Check sheet for the modelled part. Datum: model origin and axes. Units: mm. Face numbers are marked on the shaded views. A direction names the side the tool comes from. Round coordinates to 2 decimals unless told otherwise and drop trailing zeros. Order: outer loops, then holes, each group sorted by start corner. A loop starts at its lowest first (then second) coordinate and runs counter-clockwise, first axis right, second up.
Q1. Cross-section at A-A on z = 43.5. Record the cut outline in (x, y), then the cut area to 3 significant figures.
Q2. Scan lines: probe 1 along X at (y, z) = (-35, 46.5); probe 2 along Y at (x, z) = (-42, 41.25); probe 3 along X at (y, z) = (-59.5, 40.5). Record each from-to range of solid material in increasing order.
Q3. Cross-section at D-D on z = 49. Record the cut outline in (x, y).
Q4. Cross-section at C-C on y = -49. Record the cut outline in (x, z).
Q5. Set-up check for the marked faces 1 and 2: record each of +Z, -Z, +X, -X, +Y, -Y from which the full face is reachable in a straight line by a thin tool's end or side.
Q6. Cross-section at B-B on x = -55. Record the cut outline in (y, z), then the cut area to 3 significant figures.
Q7. Depth check by flat-ended pin: P1, Ø1, axis at x = -44, y = -26.5, coming from the -Z side; P2, Ø4, axis at x = -65.5, z = 44, coming from the -Y side; P3, Ø3, axis at x = -36, z = 42.5, coming from the -Y side. Enter the tip coordinate at first touch or a pass-through.
Q8. Mould release check, pull along X, two halves, no side actions. Record for the marked faces 3, 4, 5 and 6: +X half, -X half, draft (parallel to the pull), parting line (faces both ways), or undercut.
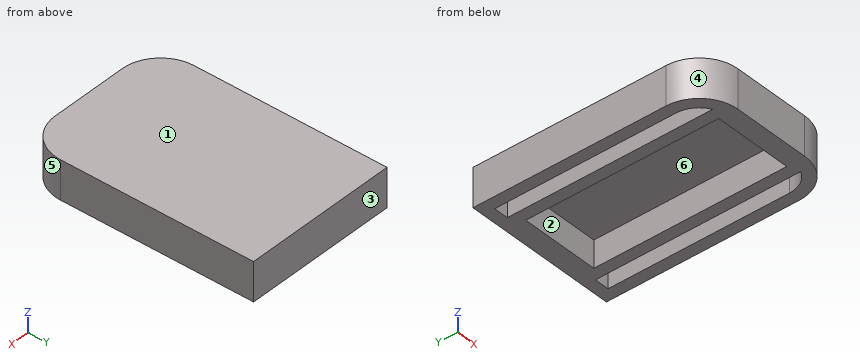
from build123d import *

# Parameters (mm, degrees)
SALIENTE_EXTRUIR1_DEPTH      = 50
CROQUIS2_W                   = 40
CROQUIS2_H                   = 50
SALIENTE_EXTRUIR2_DEPTH      = 60
SALIENTE_EXTRUIR2_DEPTH_BACK = 31
REDONDEO1_R                  = 10
REDONDEO2_R                  = 10
CORTAR_EXTRUIR1_DEPTH        = 74
VACIADO1_T                   = -3
CROQUIS4_W                   = 26.4
CROQUIS4_H                   = 56
CROQUIS4_W_2                 = 20.4
CROQUIS4_H_2                 = 50
SALIENTE_EXTRUIR3_DEPTH      = 7


with BuildPart() as part:
    # Croquis1 → Saliente-Extruir1 (new body)
    with BuildSketch(Plane.XY):
        with BuildLine():
            Line((-80.606796451, 54.173553719), (-40.606796451, 54.173553719))
            ThreePointArc((-40.606796451, 54.173553719), (-33.53572864, 51.244621531), (-30.606796451, 44.173553719))
            Line((-30.606796451, 44.173553719), (-30.606796451, 4.173553719))
            ThreePointArc((-30.606796451, 4.173553719), (-33.53572864, -2.897514093), (-40.606796451, -5.826446281))
            Line((-40.606796451, -5.826446281), (-80.606796451, -5.826446281))
            ThreePointArc((-80.606796451, -5.826446281), (-87.677864263, -2.897514093), (-90.606796451, 4.173553719))
            Line((-90.606796451, 4.173553719), (-90.606796451, 44.173553719))
            ThreePointArc((-90.606796451, 44.173553719), (-87.677864263, 51.244621531), (-80.606796451, 54.173553719))
        make_face()
    extrude(amount=SALIENTE_EXTRUIR1_DEPTH)

    # Croquis2 → Saliente-Extruir2 (add, two sides)
    with BuildSketch(Plane.XZ.offset(5.826446281)) as saliente_extruir2_sk:
        with Locations((-50.606796451, 25)):
            Rectangle(CROQUIS2_W, CROQUIS2_H)
    extrude(amount=SALIENTE_EXTRUIR2_DEPTH)
    extrude(saliente_extruir2_sk.sketch, amount=-SALIENTE_EXTRUIR2_DEPTH_BACK)

    # Redondeo1
    redondeo1_edges = [part.edges().sort_by_distance(p)[0] for p in [
        (-30.606796451, -65.826446281, 25),
    ]]
    fillet(redondeo1_edges, radius=REDONDEO1_R)

    # Redondeo2
    redondeo2_edges = [part.edges().sort_by_distance(p)[0] for p in [
        (-70.606796451, -65.826446281, 25),
    ]]
    fillet(redondeo2_edges, radius=REDONDEO2_R)

    # Croquis3 → Cortar-Extruir1 (cut)
    with BuildSketch(Plane(origin=(-30.606796451, 0, 0), x_dir=(0, 0, -1), z_dir=(1, 0, 0))):
        Polygon((-40, -65.826446281), (-40, -5.826446281), (-50, -5.826446281), (-90.954417086, -5.826446281), (-90.954417086, 59.755258828), (17.577829589, 59.755258828), (17.577829589, -73.598263991), (-40, -73.598263991), align=None)
    extrude(amount=-CORTAR_EXTRUIR1_DEPTH, mode=Mode.SUBTRACT)

    # Vaciado1
    vaciado1_openings = [part.faces().sort_by_distance(p)[0] for p in [
        (-50.606796451, -43.183468885, 40),
    ]]
    offset(amount=VACIADO1_T, openings=vaciado1_openings, kind=Kind.INTERSECTION)

    # Croquis4 → Saliente-Extruir3 (add)
    with BuildSketch(Plane(origin=(0, 0, 47), x_dir=(-1, 0, 0), z_dir=(0, 0, -1))):
        with Locations((50.606796451, -36.026446281)):
            Rectangle(CROQUIS4_W, CROQUIS4_H)
        with Locations((50.606796451, -36.026446281)):
            Rectangle(CROQUIS4_W_2, CROQUIS4_H_2, mode=Mode.SUBTRACT)
    extrude(amount=SALIENTE_EXTRUIR3_DEPTH)


solid = part.part
Results found:
1. outline: (-70.61, -55.83) arc R10 ccw to (-60.61, -65.83) - (-40.61, -65.83) arc R10 ccw to (-30.61, -55.83) - (-30.61, -5.83) - (-70.61, -5.83) - close; hole (-67.61, -55.83) arc R7 ccw to (-63.81, -62.05) - (-63.81, -8.83) - (-67.61, -8.83) - close; hole (-60.81, -61.03) - (-40.41, -61.03) - (-40.41, -11.03) - (-60.81, -11.03) - close; hole (-37.41, -62.05) arc R7 ccw to (-33.61, -55.83) - (-33.61, -8.83) - (-37.41, -8.83) - close
1. area: 946 mm2
2. probe 1: x = -70.61 to -67.61, -63.81 to -60.81, -40.41 to -37.41, -33.61 to -30.61
2. probe 2: y = -65.83 to -61.03, -11.03 to -5.83
2. probe 3: x = -69.91 to -66.57, -63.81 to -60.81, -40.41 to -37.41, -34.65 to -31.31
3. outline: (-70.61, -55.83) arc R10 ccw to (-60.61, -65.83) - (-40.61, -65.83) arc R10 ccw to (-30.61, -55.83) - (-30.61, -5.83) - (-70.61, -5.83) - close
4. outline: (-70.61, 40) - (-67.61, 40) - (-67.61, 47) - (-63.81, 47) - (-63.81, 40) - (-60.81, 40) - (-60.81, 47) - (-40.41, 47) - (-40.41, 40) - (-37.41, 40) - (-37.41, 47) - (-33.61, 47) - (-33.61, 40) - (-30.61, 40) - (-30.61, 50) - (-70.61, 50) - close
5. face 1: +Z, +X, -X, +Y, -Y
5. face 2: -Z
6. outline: (-65.83, 40) - (-61.03, 40) - (-61.03, 47) - (-11.03, 47) - (-11.03, 40) - (-5.83, 40) - (-5.83, 50) - (-65.83, 50) - close
6. area: 250 mm2
7. P1: stops at z = 47
7. P2: stops at y = -65.4
7. P3: stops at y = -65.33
8. face 3: draft
8. face 4: -X half
8. face 5: +X half
8. face 6: undercut
